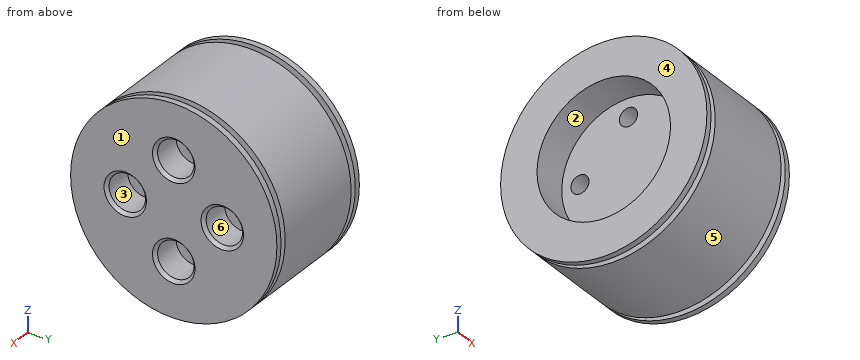
from build123d import *

# Parameters (mm, degrees)
SKETCH1_R           = 17
BOSS_EXTRUDE1_DEPTH = 1
SKETCH2_R           = 15
BOSS_EXTRUDE2_DEPTH = 1
SKETCH4_R           = 17
BOSS_EXTRUDE3_DEPTH = 16
SKETCH5_R           = 13
BOSS_EXTRUDE4_DEPTH = 1
SKETCH6_R           = 17
BOSS_EXTRUDE5_DEPTH = 1
SKETCH7_R           = 11
CUT_EXTRUDE1_DEPTH  = 6
SKETCH8_R           = 1.5
CUT_EXTRUDE2_DEPTH  = 14
SKETCH9_R           = 3
CUT_EXTRUDE3_DEPTH  = 5
CHAMFER1_SIZE       = 0.5


with BuildPart() as part:
    # Sketch1 → Boss-Extrude1 (new body)
    with BuildSketch(Plane(origin=(0, 0, 0), x_dir=(0, 0, -1), z_dir=(1, 0, 0))):
        Circle(SKETCH1_R)
    extrude(amount=BOSS_EXTRUDE1_DEPTH)

    # Sketch2 → Boss-Extrude2 (add)
    with BuildSketch(Plane(origin=(1, 0, 0), x_dir=(0, 0, -1), z_dir=(1, 0, 0))):
        Circle(SKETCH2_R)
    extrude(amount=BOSS_EXTRUDE2_DEPTH)

    # Sketch4 → Boss-Extrude3 (add)
    with BuildSketch(Plane(origin=(2, 0, 0), x_dir=(0, 0, -1), z_dir=(1, 0, 0))):
        Circle(SKETCH4_R)
    extrude(amount=BOSS_EXTRUDE3_DEPTH)

    # Sketch5 → Boss-Extrude4 (add)
    with BuildSketch(Plane(origin=(18, 0, 0), x_dir=(0, 0, -1), z_dir=(1, 0, 0))):
        Circle(SKETCH5_R)
    extrude(amount=BOSS_EXTRUDE4_DEPTH)

    # Sketch6 → Boss-Extrude5 (add)
    with BuildSketch(Plane(origin=(19, 0, 0), x_dir=(0, 0, -1), z_dir=(1, 0, 0))):
        Circle(SKETCH6_R)
    extrude(amount=BOSS_EXTRUDE5_DEPTH)

    # Sketch7 → Cut-Extrude1 (cut)
    with BuildSketch(Plane.ZY):
        Circle(SKETCH7_R)
    extrude(amount=-CUT_EXTRUDE1_DEPTH, mode=Mode.SUBTRACT)

    # Sketch8 → Cut-Extrude2 (cut)
    with BuildSketch(Plane.ZY.offset(-6)):
        with Locations((0, 8)):
            Circle(SKETCH8_R)
        with Locations((8, 0)):
            Circle(SKETCH8_R)
        with Locations((0, -8)):
            Circle(SKETCH8_R)
        with Locations((-8, 0)):
            Circle(SKETCH8_R)
    extrude(amount=-CUT_EXTRUDE2_DEPTH, mode=Mode.SUBTRACT)

    # Sketch9 → Cut-Extrude3 (cut)
    with BuildSketch(Plane(origin=(20, 0, 0), x_dir=(0, 0, -1), z_dir=(1, 0, 0))):
        with Locations((-8, 0)):
            Circle(SKETCH9_R)
        with Locations((0, 8)):
            Circle(SKETCH9_R)
        with Locations((8, 0)):
            Circle(SKETCH9_R)
        with Locations((0, -8)):
            Circle(SKETCH9_R)
    extrude(amount=-CUT_EXTRUDE3_DEPTH, mode=Mode.SUBTRACT)

    # Chamfer1
    chamfer1_edges = [part.edges().sort_by_distance(p)[0] for p in [
        (20, 0, 11),
        (20, 8, 3),
        (20, 0, -5),
        (20, -8, 3),
    ]]
    chamfer(chamfer1_edges, length=CHAMFER1_SIZE)


solid = part.part
CAD build for the part. Positions are in the model's coordinates, mm. Face numbers are marked on the shaded views. A direction names the side the tool comes from. Give positions to 0.01 mm unless a question says otherwise; leave off trailing zeros. Order: outer loops, then holes, each group sorted by start corner. A loop starts at its lowest first (then second) coordinate and runs counter-clockwise, first axis right, second up. Notation, with made-up numbers: (58, 22.5) - (97, 22.5) arc R18 cw to (97, 49.5) - close; hole circle Ø4 at (14.25, -30.5). An arc over 180 degrees is marked (long way). Answer in a Markdown table with one row per item.
1. Saw through at C-C, the plane x = 11.25. Give the cut face in (y, z), plus the area to 3 significant figures.
Data:
| item | result |
|---|---|
| outline | circle Ø34 at (0, 0); hole circle Ø3 at (-8, 0); hole circle Ø3 at (0, -8); hole circle Ø3 at (0, 8); hole circle Ø3 at (8, 0) |
| area | 880 mm² |
2. Tool access for the marked faces 1, 2 and 3: list every direction of +Z, -Z, +X, -X, +Y, -Y with a clear straight run to the whole face (end or side of a thin tool).
Data:
| item | result |
|---|---|
| face 1 | +Z, -Z, +X, +Y, -Y |
| face 2 | -X |
| face 3 | +X |
3. Saw through at D-D, the plane z = 0. Count the separate pieces of the cut face and the enclosed holes in it, plus the area to 4 significant figures.
Data:
| item | result |
|---|---|
| separate pieces | 3 |
| enclosed holes | 0 |
| area | 421.5 mm² |
4. Probe probe 1 along X at (y, z) = (11, -11); probe 2 along Y at (x, z) = (17.25, 0); probe 3 along X at (y, z) = (13, -4). List the from-to ranges inside material, lowest first. Write a range as [from, to].
Data:
| item | result |
|---|---|
| probe 1 | x = [0, 1], [2, 18], [19, 20] |
| probe 2 | y = [-17, -11], [-5, 5], [11, 17] |
| probe 3 | x = [0, 18], [19, 20] |
5. Saw through at B-B, the plane z = -13.5. Give the cut face in (x, y), plus the area to 3 significant figures.
Data:
| item | result |
|---|---|
| outline | (0, -10.33) - (1, -10.33) - (1, -6.54) - (2, -6.54) - (2, -10.33) - (18, -10.33) - (18, 10.33) - (2, 10.33) - (2, 6.54) - (1, 6.54) - (1, 10.33) - (0, 10.33) - close; (19, -10.33) - (20, -10.33) - (20, 10.33) - (19, 10.33) - close |
| area | 385 mm² |
6. Pull direction Y, two halves, no side cores. Call the marked faces 4, 5 and 6: pulls with the +Y half, pulls with the -Y half, needs draft (parallel to the pull), parting line crosses it, or undercut.
Data:
| item | result |
|---|---|
| face 4 | needs draft |
| face 5 | parting line crosses it |
| face 6 | undercut |
7. Flat gauge pins, fed straight in: pin 1 (4 mm diameter, centred on x = 13.5, y = -11, fed in from +Z); pin 2 (2.5 mm diameter, centred on y = 0, z = 8, fed in from -X); pin 3 (4 mm diameter, centred on y = 8, z = 0, fed in from -X); pin 4 (3 mm diameter, centred on y = 8.5, z = -1.5, fed in from +X). Where does each tip first touch, or does it go through?
Data:
| item | result |
|---|---|
| pin 1 | stops at z = 14.42 |
| pin 2 | passes through |
| pin 3 | stops at x = 6 |
| pin 4 | stops at x = 19.58 |
